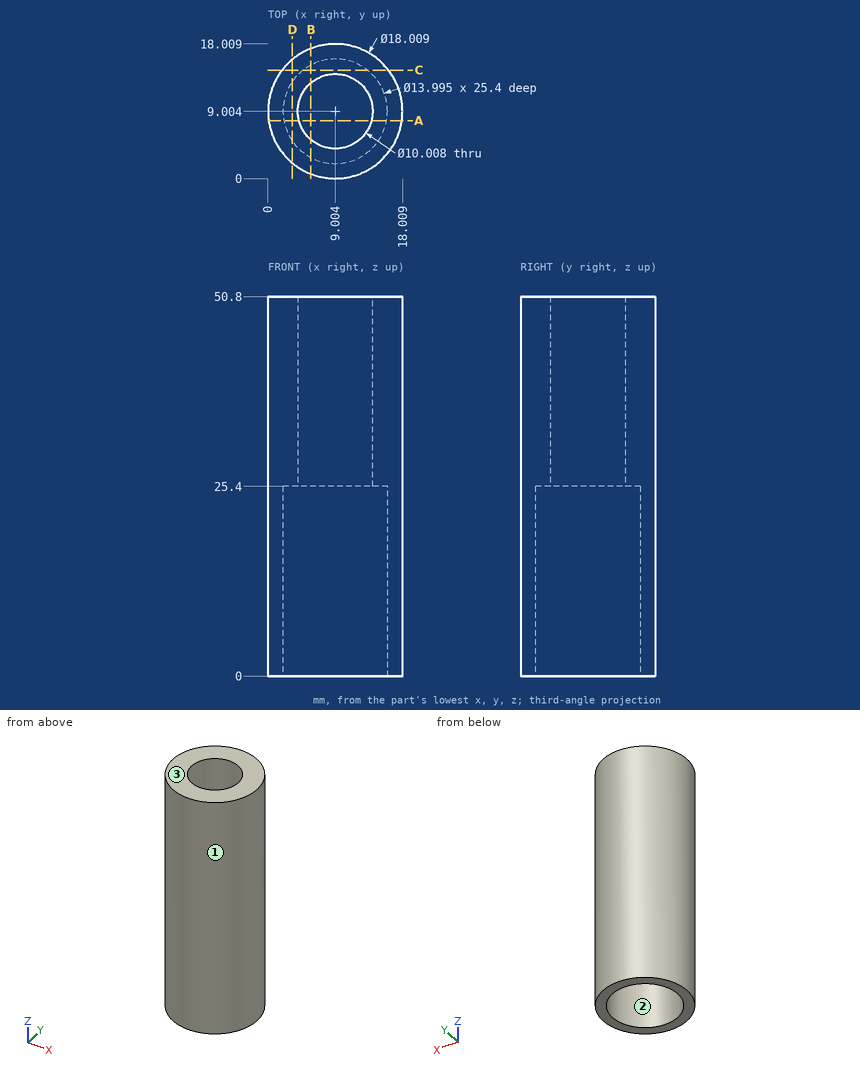
For this review, use the dimensioned drawing (mm, ordinates from the lowest corner) and the shaded views. Coordinates: 2 decimals unless noted, no trailing zeros. Loops run counter-clockwise (first coordinate to the right, second up) from the corner with the lowest first, then second, coordinate; pieces in that order, holes last. Notation, with made-up numbers: M 27.5,80 L 80.5,80 A20 ccw 80.5,109 Z; hole C 12,-36.75 d5. An arc over 180 degrees is marked long. Answer as CSV lines item,"result".
Item 1: The part is to be moulded in two halves that separate along X. For the marked faces 1, 2 and 3, say which applies: pulls with the +X half, pulls with the -X half, needs draft (parallel to the pull), parting line crosses it, or undercut.
Answer list:
face 1,"parting line crosses it"
face 2,"undercut"
face 3,"needs draft"
Item 2: For P1, Ø1.5, axis at x = 5, z = 28.5, coming from the +Y side; P2, Ø2, axis at y = 12.5, z = 15.5, coming from the +X side; P3, Ø9, axis at x = 9, y = 9, coming from the -Z side; P4, Ø6, axis at x = 5.5, z = 6, coming from the -Y side, all flat-tipped, find the tip position at first contact; note any pin that passes through.
Answer list:
P1,"y = 17.4"
P2,"x = 17.66"
P3,"through"
P4,"y = 0.01"
Item 3: For probe 1 along X at (y, z) = (8.75, 4) (1 decimal); probe 2 along Y at (x, z) = (12.25, 20) (1 decimal); probe 3 along X at (y, z) = (6.25, 12), list the stretches that pass through material, from the lowest coordinate up.
Answer list:
probe 1,"0 to 2, 16 to 18"
probe 2,"0.6 to 2.8, 15.2 to 17.4"
probe 3,"0.43 to 2.57, 15.44 to 17.58"
Item 4: Add section D-D on x = 3.25. State the section outline as (y, z) points.
Answer list:
outline,"M 2.08,0 L 5.02,0 L 5.02,25.4 L 12.99,25.4 L 12.99,0 L 15.93,0 L 15.93,50.8 L 2.08,50.8 Z"
Item 5: Add section B-B on x = 5.75. State the section outline as (y, z) points (1 decimal), plus the area to 3 significant figures.
Answer list:
outline,"M 0.6,0 L 2.8,0 L 2.8,25.4 L 5.2,25.4 L 5.2,50.8 L 0.6,50.8 Z; M 12.8,25.4 L 15.2,25.4 L 15.2,0 L 17.4,0 L 17.4,50.8 L 12.8,50.8 Z"
area,"345 mm²"
Item 6: Add section C-C on y = 14.5. State the section outline as (x, z) points.
Answer list:
outline,"M 1.87,0 L 4.67,0 L 4.67,25.4 L 13.34,25.4 L 13.34,0 L 16.14,0 L 16.14,50.8 L 1.87,50.8 Z"
Item 7: Add section A-A on y = 7.75. State the section outline as (x, z) points.
Answer list:
outline,"M 0.09,0 L 2.12,0 L 2.12,25.4 L 4.16,25.4 L 4.16,50.8 L 0.09,50.8 Z; M 13.85,25.4 L 15.89,25.4 L 15.89,0 L 17.92,0 L 17.92,50.8 L 13.85,50.8 Z"
